The model under review builds one solid part; all positions refer to its coordinate system, in mm. Face numbers are marked on the shaded views. A direction names the side the tool comes from. Give positions to 0.01 mm unless a question says otherwise; leave off trailing zeros. Loops run counter-clockwise (first coordinate to the right, second up) from the corner with the lowest first, then second, coordinate; pieces in that order, holes last. Notation, with made-up numbers: (-22, 46) - (12, 46) arc R26 cw to (12, 70) - close; hole circle Ø2 at (-37, 36). An arc over 180 degrees is marked (long way). Answer as a JSON object with one key per item and string values.
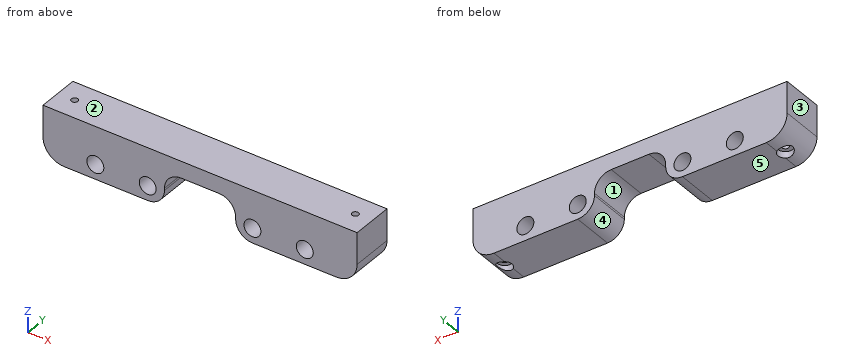
from build123d import *

# Parameters (mm, degrees)
SKETCH1_W           = 150
SKETCH1_H           = 25
SKETCH1_R           = 4.05
BOSS_EXTRUDE1_DEPTH = 20
FILLET1_R           = 10
SKETCH3_R           = 1.55
CUT_EXTRUDE1_DEPTH  = 26
SKETCH3_3_R         = 3.5
SKETCH3_3_R_2       = 1.55
CUT_EXTRUDE2_DEPTH  = 3
SKETCH4_W           = 34
SKETCH4_H           = 34.075617562
CUT_EXTRUDE3_DEPTH  = 21.0000001
FILLET2_R           = 8


with BuildPart() as part:
    # Sketch1 → Boss-Extrude1 (new body)
    with BuildSketch(Plane(origin=(0, 0, 0), x_dir=(1, 0, 0), z_dir=(0, 1, 0))):
        Rectangle(SKETCH1_W, SKETCH1_H)
        with Locations(Location((-25, 5.5, 0), (0, 0, 270))):  # turned: the seam where the file's is
            Circle(SKETCH1_R, mode=Mode.SUBTRACT)
        with Locations(Location((25, 5.5, 0), (0, 0, 270))):  # turned: the seam where the file's is
            Circle(SKETCH1_R, mode=Mode.SUBTRACT)
        with Locations(Location((-50, 5.5, 0), (0, 0, 270))):  # turned: the seam where the file's is
            Circle(SKETCH1_R, mode=Mode.SUBTRACT)
        with Locations(Location((50, 5.5, 0), (0, 0, 270))):  # turned: the seam where the file's is
            Circle(SKETCH1_R, mode=Mode.SUBTRACT)
    extrude(amount=BOSS_EXTRUDE1_DEPTH)

    # Fillet1
    fillet1_edges = [part.edges().sort_by_distance(p)[0] for p in [
        (-75, 10, -12.5),
        (75, 10, -12.5),
    ]]
    fillet(fillet1_edges, radius=FILLET1_R)

    # Sketch3 → Cut-Extrude1 (cut, through all)
    with BuildSketch(Plane(origin=(0, 0, -12.5), x_dir=(-1, 0, 0), z_dir=(0, 0, -1))):
        with Locations((-67, 10)):
            Circle(SKETCH3_R)
        with Locations((67, 10)):
            Circle(SKETCH3_R)
    extrude(amount=-CUT_EXTRUDE1_DEPTH, mode=Mode.SUBTRACT)

    # Sketch3_3 → Cut-Extrude2 (cut)
    with BuildSketch(Plane(origin=(0, 0, -12.5), x_dir=(-1, 0, 0), z_dir=(0, 0, -1))):
        with Locations((-67, 10)):
            Circle(SKETCH3_3_R)
        with Locations((-67, 10)):
            Circle(SKETCH3_3_R_2, mode=Mode.SUBTRACT)
        with Locations((67, 10)):
            Circle(SKETCH3_3_R)
        with Locations((67, 10)):
            Circle(SKETCH3_3_R_2, mode=Mode.SUBTRACT)
    extrude(amount=-CUT_EXTRUDE2_DEPTH, mode=Mode.SUBTRACT)

    # Sketch4 → Cut-Extrude3 (cut, through all)
    with BuildSketch(Plane(origin=(0, 20, 0), x_dir=(1, 0, 0), z_dir=(0, 1, 0))):
        with Locations((0, 12.5)):
            Rectangle(SKETCH4_W, SKETCH4_H)
    extrude(amount=-CUT_EXTRUDE3_DEPTH, mode=Mode.SUBTRACT)

    # Fillet2
    fillet2_edges = [part.edges().sort_by_distance(p)[0] for p in [
        (-17, 10, -12.5),
        (17, 10, -12.5),
        (-17, 10, 4.537808781),
        (17, 10, 4.537808781),
    ]]
    fillet(fillet2_edges, radius=FILLET2_R)


solid = part.part
Q1. Clearance check with flat-ended pins moving along their axes: pin 1 Ø0.8 at (y, z) = (5.5, -4) entering from +X; pin 2 Ø5 at (x, y) = (-13.5, 2) entering from -Z; pin 3 Ø2.5 at (x, y) = (67, 10) entering from -Z; pin 4 Ø1 at (y, z) = (17.5, -8.5) entering from -X. State where each tip first meets the part, or that it passes through.
Results:
{"pin 1": "stops at x = 74.94", "pin 2": "stops at z = 0.41", "pin 3": "passes through", "pin 4": "stops at x = -73.35"}
Q2. The part is to be moulded in two halves that separate along X. For the marked faces 3, 4 and 5, say which applies: +X half, -X half, draft (parallel to the pull), parting line (faces both ways), or undercut.
Results:
{"face 3": "-X half", "face 4": "undercut", "face 5": "draft"}
Q3. Consider section C-C, the plane z = -7.5. State the section outline as (x, y) points, plus the area to 3 significant figures.
Results:
{"outline": "(-73.66, 0) - (-53.52, 0) - (-53.52, 20) - (-73.66, 20) - close; (-46.48, 0) - (-28.52, 0) - (-28.52, 20) - (-46.48, 20) - close; (-21.48, 0) - (-17.58, 0) - (-17.58, 20) - (-21.48, 20) - close; (17.58, 0) - (21.48, 0) - (21.48, 20) - (17.58, 20) - close; (28.52, 0) - (46.48, 0) - (46.48, 20) - (28.52, 20) - close; (53.52, 0) - (73.66, 0) - (73.66, 20) - (53.52, 20) - close; hole circle Ø3.1 at (-67, 10); hole circle Ø3.1 at (67, 10)", "area": "1,660 mm^2"}
Q4. Consider section B-B, the plane y = 10. State how many separate pieces and enclosed holes the cut face has, plus the area to 3 significant figures.
Results:
{"separate pieces": "3", "enclosed holes": "4", "area": "2,750 mm^2"}
Q5. For the marked faces 1 and 2, list the 3-axis set-ups (+Z, -Z, +X, -X, +Y, -Y) from which the entire face can be reached by the end or side of a thin tool; tool diameter is ignored.
Results:
{"face 1": "-Z, +Y, -Y", "face 2": "+Z, +X, -X, +Y, -Y"}
Q6. Consider section A-A, the plane x = 50. State the section outline as (y, z) points, plus the area to 3 significant figures.
Results:
{"outline": "(0, -12.5) - (20, -12.5) - (20, -9.55) - (0, -9.55) - close; (0, -1.45) - (20, -1.45) - (20, 12.5) - (0, 12.5) - close", "area": "338 mm^2"}
Q7. To check wall thickness, follow probe 1 along Y at (x, z) = (67, 2.5); probe 2 along X at (y, z) = (12.25, -5.5); probe 3 along X at (y, z) = (9.5, 1.75). State the ranges of each line that lie inside material, in increasing order. Write a range as [from, to].
Results:
{"probe 1": "y = [0, 8.45], [11.55, 20]", "probe 2": "x = [-74.54, -54.05], [-45.95, -29.05], [-20.95, -17.06], [17.06, 20.95], [29.05, 45.95], [54.05, 74.54]", "probe 3": "x = [-75, -68.47], [-65.53, -15.07], [15.07, 65.53], [68.47, 75]"}
Q8. Consider section D-D, the plane x = -67. State the section outline as (y, z) points.
Results:
{"outline": "(0, -12.3) - (6.5, -12.3) - (6.5, -9.5) - (8.45, -9.5) - (8.45, 12.5) - (0, 12.5) - close; (11.55, -9.5) - (13.5, -9.5) - (13.5, -12.3) - (20, -12.3) - (20, 12.5) - (11.55, 12.5) - close"}
